from build123d import *

# Parameters (mm, degrees)
ESTRUSIONE_ESTRUSIONE1_DEPTH = 10
SCHIZZO5_R                   = 1.625
SCHIZZO5_R_2                 = 1.5
TAGLIO_ESTRUSIONE1_DEPTH     = 10
SCHIZZO6_R                   = 3.5
TAGLIO_ESTRUSIONE2_DEPTH     = 2
TAGLIO_ESTRUSIONE3_START     = -8
SCHIZZO6_2_R                 = 3.5
TAGLIO_ESTRUSIONE3_DEPTH     = 12
TAGLIO_ESTRUSIONE4_START     = -2
SCHIZZO7_R                   = 3.5
TAGLIO_ESTRUSIONE4_DEPTH     = 6
RACCORDO1_R                  = 2
RACCORDO2_R                  = 2


with BuildPart() as part:
    # Schizzo1 → Estrusione-Estrusione1 (new body)
    with BuildSketch(Plane.XY):
        with BuildLine():
            Line((-24.824967097, 11.313668705), (-10.824967097, 11.313668705))
            ThreePointArc((-10.824967097, 11.313668705), (-9.092916289, 5.864178962), (-13.653394221, 9.313668705))
            Line((-13.653394221, 9.313668705), (-21.996539972, 9.313668705))
            ThreePointArc((-21.996539972, 9.313668705), (-26.557017904, 5.864178962), (-24.824967097, 11.313668705))
        make_face()
    extrude(amount=ESTRUSIONE_ESTRUSIONE1_DEPTH)

    # Schizzo5 → Taglio-Estrusione1 (cut)
    with BuildSketch(Plane(origin=(0, 0, 0), x_dir=(-1, 0, 0), z_dir=(0, 0, -1))):
        with Locations((10.824967097, 8.313668705)):
            Circle(SCHIZZO5_R)
        with Locations((24.824967097, 8.313668705)):
            Circle(SCHIZZO5_R_2)
    extrude(amount=-TAGLIO_ESTRUSIONE1_DEPTH, mode=Mode.SUBTRACT)

    # Schizzo6 → Taglio-Estrusione2 (cut)
    with BuildSketch(Plane(origin=(0, 0, 0), x_dir=(-1, 0, 0), z_dir=(0, 0, -1))):
        with Locations((24.824967097, 8.313668705)):
            Circle(SCHIZZO6_R)
    extrude(amount=-TAGLIO_ESTRUSIONE2_DEPTH, mode=Mode.SUBTRACT)

    # Schizzo6<2> → Taglio-Estrusione3 (cut)
    with BuildSketch(Plane(origin=(0, 0, 0), x_dir=(-1, 0, 0), z_dir=(0, 0, -1)).offset(TAGLIO_ESTRUSIONE3_START)):
        with Locations((24.824967097, 8.313668705)):
            Circle(SCHIZZO6_2_R)
    extrude(amount=-TAGLIO_ESTRUSIONE3_DEPTH, mode=Mode.SUBTRACT)

    # Schizzo7 → Taglio-Estrusione4 (cut)
    with BuildSketch(Plane(origin=(0, 0, 0), x_dir=(-1, 0, 0), z_dir=(0, 0, -1)).offset(TAGLIO_ESTRUSIONE4_START)):
        with Locations((10.824967097, 8.313668705)):
            Circle(SCHIZZO7_R)
    extrude(amount=-TAGLIO_ESTRUSIONE4_DEPTH, mode=Mode.SUBTRACT)

    # Raccordo1
    raccordo1_edges = [part.edges().sort_by_distance(p)[0] for p in [
        (-21.996539972, 9.313668705, 5),
    ]]
    fillet(raccordo1_edges, radius=RACCORDO1_R)

    # Raccordo2
    raccordo2_edges = [part.edges().sort_by_distance(p)[0] for p in [
        (-13.653394221, 9.313668705, 1),
    ]]
    fillet(raccordo2_edges, radius=RACCORDO2_R)


solid = part.part
Geometry: final body of the model. Coordinates: model frame, mm. A direction names the side the tool comes from. Give positions to 0.01 mm unless a question says otherwise; leave off trailing zeros. Order: outer loops, then holes, each group sorted by start corner. A loop starts at its lowest first (then second) coordinate and runs counter-clockwise, first axis right, second up. Notation, with made-up numbers: (37, -36) -> (77, -36) arc R30 ccw to (77, -2) -> close; hole circle Ø6 at (1.5, -20.75). An arc over 180 degrees is marked (long way). Write each question's results on one line, items separated by ' | '.
1) Set-up query: faces 4 (the face through (-21.896, 10.23, 0.986)), 5 (the face through (-18, 9.314, 5)), 6 (the face through (-24, 10, 8)). Return all of +Z, -Z, +X, -X, +Y, -Y with unobstructed straight access to the full face (end or side cutting, diameter ignored); none if empty.
Geometry says:
face 4: -Z, -X, -Y | face 5: +Z, -Z, -Y | face 6: +Z, -X, -Y
2) Cut plane D-D (x = -16.75). Output: boundary loops of the cut face in (y, z), and give its area (3 significant figures).
Geometry says:
outline: (9.31, 0) -> (11.31, 0) -> (11.31, 10) -> (9.31, 10) -> close | area: 20.0 mm²
3) Draft query along X for faces 1 (the face through (-8.442, 6.491, 8.986)), 2 (the face through (-12, 10, 8)), 3 (the face through (-21, 9, 5)). Return one class per face: released by +X, released by -X, zero draft, split by the parting line, or undercut.
Geometry says:
face 1: split by the parting line | face 2: zero draft | face 3: undercut
4) Cut plane C-C (y = 7.9). Output: boundary loops of the cut face in (x, z), and give its area (3 significant figures).
Geometry says:
outline: (-27.8, 2) -> (-26.27, 2) -> (-26.27, 8) -> (-27.8, 8) -> close; (-23.38, 2) -> (-21.84, 2) -> (-21.84, 8) -> (-23.38, 8) -> close; (-13.81, 0) -> (-12.4, 0) -> (-12.4, 2) -> (-13.81, 2) -> close; (-13.81, 8) -> (-12.4, 8) -> (-12.4, 10) -> (-13.81, 10) -> close; (-9.25, 0) -> (-7.85, 0) -> (-7.85, 2) -> (-9.25, 2) -> close; (-9.25, 8) -> (-7.85, 8) -> (-7.85, 10) -> (-9.25, 10) -> close | area: 29.7 mm²
5) Cut plane A-A (z = 5.5). Output: boundary loops of the cut face in (x, y).
Geometry says:
outline: (-24.82, 11.31) arc R3 ccw (long way) to (-21.89, 7.71) arc R2 cw to (-19.93, 9.31) -> (-15.72, 9.31) arc R2 cw to (-14.3, 8.72) arc R3.5 cw to (-12.63, 11.31) -> close; hole circle Ø3 at (-24.82, 8.31)
6) Cut plane B-B (y = 9.1). Output: boundary loops of the cut face in (x, z), and give its area (3 significant figures).
Geometry says:
outline: (-27.72, 2) -> (-26.1, 2) -> (-26.1, 8) -> (-27.72, 8) -> close; (-23.55, 2) -> (-21.41, 2) -> (-21.41, 0) -> (-20.83, 0) -> (-20.83, 10) -> (-21.41, 10) -> (-21.41, 8) -> (-23.55, 8) -> close; (-14.82, 0) -> (-12.25, 0) -> (-12.25, 2) -> (-14.24, 2) -> (-14.24, 8) -> (-12.25, 8) -> (-12.25, 10) -> (-14.82, 10) -> close; (-9.4, 0) -> (-7.93, 0) -> (-7.93, 2) -> (-9.4, 2) -> close; (-9.4, 8) -> (-7.93, 8) -> (-7.93, 10) -> (-9.4, 10) -> close | area: 48.1 mm²
7) Line query: line 1 along X through (y, z) = (8.85, 1.5); line 2 along Z through (x, y) = (-9.5, 7.3); line 3 along Z through (x, y) = (-25.5, 10.25). Output: solid intervals per line, ascending.
Geometry says:
line 1: x = -21.37 to -21.21, -14.44 to -12.36, -9.29 to -7.87 | line 2: z = 0 to 2, 8 to 10 | line 3: z = 2 to 8
8) First-contact query: pin 1 Ø4.5 at (x, z) = (-18.5, 5) entering from -Y; pin 2 Ø3 at (x, y) = (-24, 9) entering from +Z; pin 3 Ø2 at (y, z) = (10, 5.5) entering from -X. Flat tips, straight axial feed; report the tip coordinate or a pass-through.
Geometry says:
pin 1: stops at y = 9.14 | pin 2: stops at z = 8 | pin 3: stops at x = -27.75
